Model file for the job. Use its own axes, mm. Coordinates: 2 decimals unless noted, no trailing zeros. Order: outer loops, then holes, each group sorted by start corner. A loop starts at its lowest first (then second) coordinate and runs counter-clockwise, first axis right, second up. Notation, with made-up numbers: (51.25, 2.5) - (67.25, 2.5) arc R16 ccw to (67.25, 33.5) - close; hole circle Ø10 at (-36.5, 76.5). An arc over 180 degrees is marked (long way). Put each result on its own line as item: value. Start each with the question number.
```python
from build123d import *

# Parameters (mm, degrees)
EXTRUDE_3_DEPTH          = 24
CUT_EXTRUDE_1_DEPTH      = 35.805893516
CUT_EXTRUDE_1_DEPTH_BACK = 35.805893516
SKETCH_4_R               = 2


with BuildPart() as part:
    # 草图1 → 凸台-拉伸3 (new body)
    with BuildSketch(Plane.XY):
        with BuildLine():
            Line((0, 10), (0, 0))
            ThreePointArc((0, 0), (2.928932188, 7.071067812), (10, 10))
            Line((10, 10), (10, 15.34438736))
            Line((10, 15.34438736), (5, 15.34438736))
            Line((5, 15.34438736), (0, 10))
        make_face()
        with BuildLine():
            ThreePointArc((10, 10), (17.071067812, 7.071067812), (20, 0))
            Line((20, 0), (20, 10))
            Line((20, 10), (15, 15.34438736))
            Line((15, 15.34438736), (10, 15.34438736))
            Line((10, 15.34438736), (10, 10))
        make_face()
        with BuildLine():
            ThreePointArc((10, 10), (2.928932188, 7.071067812), (0, 0))
            Line((0, 0), (10, 0))
            Line((10, 0), (10, 10))
        make_face()
        with BuildLine():
            Line((10, 10), (10, 0))
            Line((10, 0), (20, 0))
            ThreePointArc((20, 0), (17.071067812, 7.071067812), (10, 10))
        make_face()
        with BuildLine():
            Line((10, 0), (0, 0))
            ThreePointArc((0, 0), (10, -10), (20, 0))
            Line((20, 0), (10, 0))
        make_face()
    extrude(amount=EXTRUDE_3_DEPTH)

    # 草图4 → 切除-拉伸1 (cut, two sides: drawn at the far end of the back side and taken through both)
    with BuildSketch(Plane(origin=(20, 0, 0), x_dir=(0, 0, -1), z_dir=(1, 0, 0)).offset(-CUT_EXTRUDE_1_DEPTH_BACK)):
        with Locations((-20, 5)):
            Circle(SKETCH_4_R)
        with Locations((-4, 5)):
            Circle(SKETCH_4_R)
    extrude(amount=CUT_EXTRUDE_1_DEPTH + CUT_EXTRUDE_1_DEPTH_BACK, mode=Mode.SUBTRACT)


solid = part.part
```
Item 1: Flat gauge pins, fed straight in: pin 1 Ø3 at (x, z) = (12.5, 18) entering from -Y; pin 2 Ø1.5 at (x, z) = (11.5, 19.5) entering from -Y. Where does each tip first touch, or does it go through?
Item 2: Wall check: line 1 along Z through (x, y) = (9.5, 5); line 2 along Z through (x, y) = (15.75, 3.5); line 3 along Y through (x, z) = (10, 21.25). Give the ranges that are in metal, low to high.
Item 3: Slice it at B-B, the plane z = 4. Give the cut face in (x, y).
Item 4: Pull direction Z, two halves, no side cores. Call faces 1 (the face through (2.535, 12.71, 11.832)), 2 (the face through (10, 5, 22)), 3 (the face through (10, 3, 24)), 4 (the face through (10, 5, 6)): pulls with the +Z half, pulls with the -Z half, needs draft (parallel to the pull), parting line crosses it, or undercut.
Item 5: Slice it at D-D, the plane y = 12. Give the cut face in (x, z).
Item 6: Slice it at C-C, the plane x = 10. Give the cut face in (y, z), plus the area to 3 significant figures.
Item 7: Slice it at A-A, the plane y = 5. Give the cut face in (x, z), plus the area to 3 significant figures.
Here are the results:
1. pin 1: stops at y = -9.95
1. pin 2: stops at y = -9.97
2. line 1: z = 0 to 2, 6 to 18, 22 to 24
2. line 2: z = 0 to 2.68, 5.32 to 18.68, 21.32 to 24
2. line 3: y = -10 to 3.44, 6.56 to 15.34
3. outline: (0, 0) arc R10 ccw to (20, 0) - (20, 3) - (0, 3) - close; (0, 7) - (20, 7) - (20, 10) - (15, 15.34) - (5, 15.34) - (0, 10) - close
4. face 1: needs draft
4. face 2: undercut
4. face 3: pulls with the +Z half
4. face 4: undercut
5. outline: (1.87, 0) - (18.13, 0) - (18.13, 24) - (1.87, 24) - close
6. outline: (-10, 0) - (15.34, 0) - (15.34, 24) - (-10, 24) - close; hole circle Ø4 at (5, 4); hole circle Ø4 at (5, 20)
6. area: 583 mm^2
7. outline: (0, 0) - (20, 0) - (20, 2) - (0, 2) - close; (0, 6) - (20, 6) - (20, 18) - (0, 18) - close; (0, 22) - (20, 22) - (20, 24) - (0, 24) - close
7. area: 320 mm^2
